```python
from build123d import *

# Parameters (mm, degrees)
F0_W     = 37
F0_H     = 33
F1_DEPTH = 1


with BuildPart() as f1:
    # F0 (on Top) → F1 (new body)
    with BuildSketch(Plane.XY):
        Polygon((-35.418198, 50.5), (-36.418198, 50.5), (-36.418198, 17.5), (-73.418198, 17.5), (-73.418198, 16.5), (-36.418198, 16.5), (-36.418198, -16.5), (-73.418198, -16.5), (-73.418198, -17.5), (-36.418198, -17.5), (-36.418198, -50.5), (-35.418198, -50.5), (-35.418198, -17.5), (1.581802, -17.5), (1.581802, -50.5), (2.581802, -50.5), (2.581802, -17.5), (39.581802, -17.5), (39.581802, -50.5), (40.581802, -50.5), (40.581802, -17.5), (77.581802, -17.5), (77.581802, -16.5), (40.581802, -16.5), (40.581802, 16.5), (77.581802, 16.5), (77.581802, 17.5), (40.581802, 17.5), (40.581802, 50.5), (39.581802, 50.5), (39.581802, 17.5), (2.581802, 17.5), (2.581802, 50.5), (1.581802, 50.5), (1.581802, 17.5), (-35.418198, 17.5), align=None)
        with Locations((-16.918198, 0)):
            Rectangle(F0_W, F0_H, mode=Mode.SUBTRACT)
        with Locations((21.081802, 0)):
            Rectangle(F0_W, F0_H, mode=Mode.SUBTRACT)
    extrude(amount=F1_DEPTH)


solid = f1.part
```
The listing builds one solid part. Answer for the finished solid, in the listing's coordinates (mm). Give positions to 0.01 mm unless a question says otherwise; leave off trailing zeros. Order: outer loops, then holes, each group sorted by start corner. A loop starts at its lowest first (then second) coordinate and runs counter-clockwise, first axis right, second up. Notation, with made-up numbers: (76.5, 39.25) -> (86.5, 39.25) arc R29 ccw to (86.5, 73.25) -> close; hole circle Ø8 at (16, 67.5). An arc over 180 degrees is marked (long way). Answer as a JSON object with one key per item and string values. Group by question number.
Item 1: The part is cut by section B-B on y = -36. Write down the section's boundary in (x, z), and give its area (3 significant figures).
Item 2: Consider L1, parallel to X at y = -23, z = 0.5; L2, parallel to Y at x = -50, z = 0.85. Determine where each line is inside the solid, lowest interval first. Write a range as from..to.
Item 3: Flat-ended cylindrical pins translate along their axes: pin 1 (0.5 mm diameter, centred on y = -27.5, z = 0.5, fed in from -X); pin 2 (0.5 mm diameter, centred on x = 20, z = 0.5, fed in from -Y); pin 3 (0.5 mm diameter, centred on x = -60, z = 0.5, fed in from +Y). Find the tip coordinate at first contact, or state that the pin passes through.
Item 4: The part is cut by section A-A on x = -42.5. Write down the section's boundary in (y, z), and give its area (3 significant figures).
Item 5: The part is cut by section C-C on z = 0.25. Give the number of separate pieces and of enclosed holes in the cut face, and give its area (3 significant figures).
Result set:
{
 "1": {"outline": "(-36.42, 0) -> (-35.42, 0) -> (-35.42, 1) -> (-36.42, 1) -> close; (1.58, 0) -> (2.58, 0) -> (2.58, 1) -> (1.58, 1) -> close; (39.58, 0) -> (40.58, 0) -> (40.58, 1) -> (39.58, 1) -> close", "area": "3.00 mm²"},
 "2": {"L1": "-36.42..-35.42, 1.58..2.58, 39.58..40.58", "L2": "-17.5..-16.5, 16.5..17.5"},
 "3": {"pin 1": "x = -36.42", "pin 2": "y = -17.5", "pin 3": "y = 17.5"},
 "4": {"outline": "(-17.5, 0) -> (-16.5, 0) -> (-16.5, 1) -> (-17.5, 1) -> close; (16.5, 0) -> (17.5, 0) -> (17.5, 1) -> (16.5, 1) -> close", "area": "2.00 mm²"},
 "5": {"separate pieces": "1", "enclosed holes": "2", "area": "599 mm²"}
}
